Can you work these out from the model? Positions are in its coordinate system, mm. Face numbers are marked on the shaded views. A direction names the side the tool comes from. Give positions to 0.01 mm unless a question says otherwise; leave off trailing zeros. Order: outer loops, then holes, each group sorted by start corner. A loop starts at its lowest first (then second) coordinate and runs counter-clockwise, first axis right, second up. Notation, with made-up numbers: (60, 69) - (109, 69) arc R20 ccw to (109, 86) - close; hole circle Ø9 at (38, -34). An arc over 180 degrees is marked (long way). Answer as CSV lines item,"result".
```python
from build123d import *

# Parameters (mm, degrees)
F0_W      = 38.1
F0_H      = 38.099996
F1_DEPTH  = 38.1
F6_DEPTH  = 38.1
F8_DEPTH  = 38.1
F9_W      = 25.4
F9_H      = 7.62
F10_DEPTH = 38.1


with BuildPart() as f1:
    # F0 (on Front) → F1 (new body)
    with BuildSketch(Plane.XZ):
        with Locations((19.05, 19.049998)):
            Rectangle(F0_W, F0_H)
    extrude(amount=F1_DEPTH)

    # F5 (on offset) → F6 (cut)
    with BuildSketch(Plane.YZ.offset(38.1)):
        Polygon((-31.75, 0), (-38.1, 38.1), (-38.1, 0), align=None)
        Polygon((-11.43, 18.195421), (-6.35, 38.1), (-31.75, 38.1), (-26.67, 18.195421), (-21.59, 30.895421), (-16.51, 30.895421), align=None)
        Polygon((-25.4, 0), (-12.7, 0), (-19.05, 15.875), align=None)
        Polygon((-6.35, 0), (0, 0), (0, 38.1), align=None)
    extrude(amount=-F6_DEPTH, mode=Mode.SUBTRACT)

    # F7 (on offset) → F8 (cut)
    with BuildSketch(Plane.XZ.offset(38.1)):
        Polygon((0, 38.1), (0, 0), (6.35, 38.1), align=None)
        Polygon((25.4, 38.1), (12.7, 38.1), (19.05, 22.225), align=None)
        Polygon((31.75, 38.1), (38.1, 0), (38.1, 38.1), align=None)
        Polygon((11.43, 22.225), (6.35, 0), (31.75, 0), (26.67, 22.225), (21.59, 9.525), (16.51, 9.525), align=None)
    extrude(amount=-F8_DEPTH, mode=Mode.SUBTRACT)

    # F9 (on offset) → F10 (cut)
    with BuildSketch(Plane.XY.offset(38.1)):
        with Locations((12.7, -26.67)):
            Rectangle(F9_W, F9_H)
        with Locations((25.4, -11.43)):
            Rectangle(F9_W, F9_H)
    extrude(amount=-F10_DEPTH, mode=Mode.SUBTRACT)


solid = f1.part
```
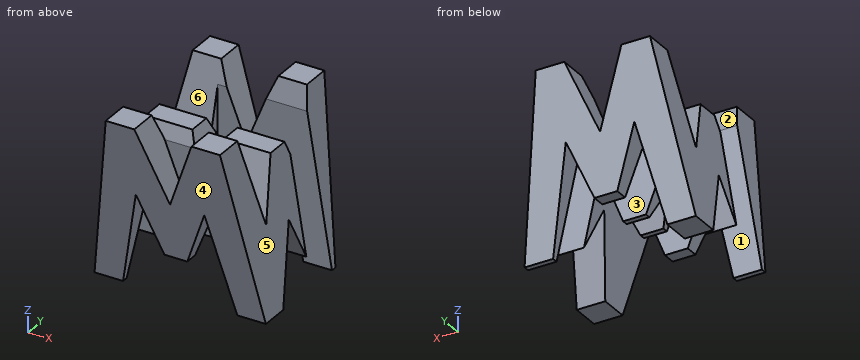
1) Which directions (+Z, -Z, +X, -X, +Y, -Y) give clear straight access to the entire face, cutting with the end or side of a thin tool? Please do the marked faces 1, 2 and 3.
Answer block:
face 1,"+Z, -Z, -X"
face 2,"+Z, +X, -X"
face 3,"+Z, -Z, +X"
2) I want a section at D-D on z = 34.5. Write out the boundary of the cut face in (x, y), plus the area to 3 significant figures.
Answer block:
outline,"(5.75, -37.5) - (14.14, -37.5) - (14.14, -30.83) - (5.75, -30.83) - close; (5.75, -7.27) - (14.14, -7.27) - (14.14, -0.6) - (5.75, -0.6) - close; (23.96, -37.5) - (32.35, -37.5) - (32.35, -30.83) - (23.96, -30.83) - close; (23.96, -7.27) - (32.35, -7.27) - (32.35, -0.6) - (23.96, -0.6) - close"
area,"224 mm2"
3) If we mould it in two halves opening along Y, with no side actions, what happens to the marked faces 4, 5 and 6? For each: +Y half, -Y half, draft (parallel to the pull), parting line (faces both ways), or undercut.
Answer block:
face 4,"-Y half"
face 5,"draft"
face 6,"undercut"
4) I want a section at C-C on x = 34.5. Write out the boundary of the cut face in (y, z) (3 decimals), plus the area to 3 significant figures.
Answer block:
outline,"(-35.35, 21.6) - (-31.75, 0) - (-25.4, 0) - (-19.05, 15.875) - (-15.24, 6.35) - (-15.24, 21.6) - (-25.308, 21.6) - (-26.67, 18.195) - (-27.539, 21.6) - close; (-7.62, 0) - (-6.35, 0) - (-2.75, 21.6) - (-7.62, 21.6) - close"
area,"365 mm2"
5) I need wall thicknesses on line 1 along Y through (x, z) = (23, 30); line 2 along Y through (x, z) = (22.5, 14); line 3 along Y through (x, z) = (25.5, 29.5). Which ranges of each line are inside material? Lowest first, please. Write a range as [from, to].
Answer block:
line 1,"[-36.75, -30.48], [-21.95, -16.15], [-7.62, -1.35]"
line 2,"[-34.08, -30.48], [-22.86, -19.8], [-18.3, -15.24], [-7.62, -4.02]"
line 3,"[-36.67, -29.56], [-22.15, -15.95], [-7.62, -1.43]"
6) I want a section at A-A on z = 30. Write out the boundary of the cut face in (x, y).
Answer block:
outline,"(5, -36.75) - (15.94, -36.75) - (15.94, -30.48) - (5, -30.48) - close; (5, -21.95) - (15.94, -21.95) - (15.94, -16.15) - (5, -16.15) - close; (5, -8.42) - (12.7, -8.42) - (12.7, -7.62) - (15.94, -7.62) - (15.94, -1.35) - (5, -1.35) - close; (22.16, -36.75) - (33.1, -36.75) - (33.1, -29.68) - (25.4, -29.68) - (25.4, -30.48) - (22.16, -30.48) - close; (22.16, -21.95) - (33.1, -21.95) - (33.1, -16.15) - (22.16, -16.15) - close; (22.16, -7.62) - (33.1, -7.62) - (33.1, -1.35) - (22.16, -1.35) - close"
7) I'm going to push flat-ended pins straight in: P1, Ø1.5, axis at x = 8, z = 14, coming from the -Y side; P2, Ø1.5, axis at x = 27, y = -18, coming from the +Z side; P3, Ø17, axis at x = 15.5, z = 17.5, coming from the -Y side. Where does each tip first touch, or does it pass through?
Answer block:
P1,"y = -34.21"
P2,"z = 30.9"
P3,"y = -36.08"
8) I want a section at B-B on x = 20.5. Count the separate pieces of the cut face and the enclosed holes in it, plus the area to 3 significant figures.
Answer block:
separate pieces,"3"
enclosed holes,"0"
area,"246 mm2"
